Input: part model. Units: mm. Frame: model coordinates. A direction names the side the tool comes from. Coordinates: 2 decimals unless noted, no trailing zeros. Write each loop counter-clockwise with the first axis right and the second up, starting at its lowest first coordinate (ties: lowest second). Pieces come first, ordered by that corner, then holes. Notation, with made-up numbers: (10.5, 18.25) - (28.5, 18.25) arc R9 ccw to (28.5, 32.25) - close; hole circle Ø11 at (9.25, -39). An arc over 180 degrees is marked (long way). One line per question, with ' | ' between items. Start each with the question number.
1) Section query C-C on y = -62.5. Return loops of the section in (x, z), and give its area (3 significant figures).
2) First-contact query: P1, Ø1.5, axis at y = 20.5, z = -8.5, coming from the +X side; P2, Ø3, axis at y = -12, z = -6.5, coming from the -X side; P3, Ø1, axis at y = 55, z = -4, coming from the +X side. Flat tips, straight axial feed; report the tip coordinate or a pass-through.
3) Draft query along X for faces 3 (the cylindrical face through (-57.423, 31.395, -5.916)), 4 (the flat face through (15, -47, 0)), 5 (the cylindrical face through (69.15, 21.78, -5.92)). Return one class per face: released by +X, released by -X, zero draft, split by the parting line, or undercut.
4) Section query B-B on x = 0. Return loops of the section in (y, z).
5) Reachability of faces 1 (the cylindrical face through (0.43, 59.23, -5.92)), 2 (the cylindrical face through (-10.3, -46.37, -0.99)) from +Z, -Z, +X, -X, +Y, -Y: full face, straight path, thin tool, end or side. Return the list, or none.
6) Line query: line 1 (Y direction, x = 0, z = -8); line 2 (Y direction, x = 0, z = -1.05); line 3 (Z direction, x = -34, y = -32.5). Output: solid intervals per line, ascending.
7) Section query A-A on y = 0. Return loops of the section in (x, z), and give its area (3 significant figures).
```python
from build123d import *

# Parameters (mm, degrees)
SKETCH1_R            = 72.5
SKETCH1_R_2          = 30
BOSS_EXTRUDE1_DEPTH  = 12
M6_CLEARANCE_HOLE1_D = 6.6
CIRPATTERN1_COUNT    = 6
SKETCH4_R            = 47.5
CUT_EXTRUDE1_DEPTH   = 2
CHAMFER1_SIZE        = 3


with BuildPart() as part:
    # Sketch1 → Boss-Extrude1 (new body)
    with BuildSketch(Plane.XY):
        Circle(SKETCH1_R)
        Circle(SKETCH1_R_2, mode=Mode.SUBTRACT)
    extrude(amount=-BOSS_EXTRUDE1_DEPTH)

    # M6 Clearance Hole1 (through all)
    with Locations(Plane(origin=(9.54608016, 92.530972723, -12), x_dir=(1, 0, 0), z_dir=(0, 0, -1))):
        with Locations((-9.54608016, 30.030972723)):
            m6_clearance_hole1 = Hole(M6_CLEARANCE_HOLE1_D / 2)

    # CirPattern1: M6 Clearance Hole1 ×6 about axis
    cirpattern1_axis = Axis((0, 0, 0), (0, 0, 1))
    for i in range(1, CIRPATTERN1_COUNT):
        add(m6_clearance_hole1.rotate(cirpattern1_axis, i * 360 / CIRPATTERN1_COUNT), mode=Mode.SUBTRACT)

    # Sketch4 → Cut-Extrude1 (cut)
    with BuildSketch(Plane.XY):
        Circle(SKETCH4_R)
    extrude(amount=-CUT_EXTRUDE1_DEPTH, mode=Mode.SUBTRACT)

    # Chamfer1
    chamfer1_edges = [part.edges().sort_by_distance(p)[0] for p in [
        (-30, 0, -2),
    ]]
    chamfer(chamfer1_edges, length=CHAMFER1_SIZE)


solid = part.part
```
Answer key:
1) outline: (-36.74, -12) - (-3.3, -12) - (-3.3, 0) - (-36.74, 0) - close; (3.3, -12) - (36.74, -12) - (36.74, 0) - (3.3, 0) - close | area: 803 mm²
2) P1: x = 69.76 | P2: x = -71.74 | P3: x = 47.81
3) face 3: undercut | face 4: zero draft | face 5: split by the parting line
4) outline: (-72.5, -12) - (-65.8, -12) - (-65.8, 0) - (-72.5, 0) - close; (-59.2, -12) - (-30, -12) - (-30, -5) - (-33, -2) - (-47.5, -2) - (-47.5, 0) - (-59.2, 0) - close; (30, -12) - (59.2, -12) - (59.2, 0) - (47.5, 0) - (47.5, -2) - (33, -2) - (30, -5) - close; (65.8, -12) - (72.5, -12) - (72.5, 0) - (65.8, 0) - close
5) face 1: +Z, -Z | face 2: +Z
6) line 1: -72.5 to -65.8, -59.2 to -30, 30 to 59.2, 65.8 to 72.5 | line 2: -72.5 to -65.8, -59.2 to -47.5, 47.5 to 59.2, 65.8 to 72.5 | line 3: -12 to -2
7) outline: (-72.5, -12) - (-30, -12) - (-30, -5) - (-33, -2) - (-47.5, -2) - (-47.5, 0) - (-72.5, 0) - close; (30, -12) - (72.5, -12) - (72.5, 0) - (47.5, 0) - (47.5, -2) - (33, -2) - (30, -5) - close | area: 941 mm²
